Geometry check sheet. Reference: the model listing, model coordinates, mm. A direction names the side the tool comes from. Give positions to 0.01 mm unless a question says otherwise; leave off trailing zeros. Loops run counter-clockwise (first coordinate to the right, second up) from the corner with the lowest first, then second, coordinate; pieces in that order, holes last. Notation, with made-up numbers: (81.25, -6) -> (106.25, -6) arc R23 ccw to (106.25, 15) -> close; hole circle Ø10 at (71, -16.5). An arc over 180 degrees is marked (long way). Answer as a JSON object with one key per item and string values.
from build123d import *

# Parameters (mm, degrees)
EXTRUDE_1_DEPTH     = 60
SKETCH_2_W          = 50
SKETCH_2_H          = 85
CUT_EXTRUDE_1_DEPTH = 70
SKETCH_3_R          = 10
CUT_EXTRUDE_2_DEPTH = 105.880884817
SKETCH_4_R          = 27.5
CUT_EXTRUDE_3_DEPTH = 107.066017178


with BuildPart() as part:
    # Эскиз1 → Бобышка-Вытянуть1 (new, symmetric)
    with BuildSketch(Plane.XY):
        Polygon((50, -25), (0, 45), (-25, 45), (-25, -25), (-50, -25), (-50, -45), (50, -45), align=None)
    extrude(amount=EXTRUDE_1_DEPTH, both=True)

    # Эскиз2 → Вырез-Вытянуть1 (cut)
    with BuildSketch(Plane(origin=(0, 45, 0), x_dir=(1, 0, 0), z_dir=(0, 1, 0))):
        with Locations((25, 0)):
            Rectangle(SKETCH_2_W, SKETCH_2_H)
    extrude(amount=-CUT_EXTRUDE_1_DEPTH, mode=Mode.SUBTRACT)

    # Эскиз3 → Вырез-Вытянуть2 (cut, through all)
    with BuildSketch(Plane(origin=(0, -25, 0), x_dir=(1, 0, 0), z_dir=(0, 1, 0))):
        with Locations(Location((25, 0, 0), (0, 0, 180))):
            Circle(SKETCH_3_R)
    extrude(amount=-CUT_EXTRUDE_2_DEPTH, mode=Mode.SUBTRACT)

    # Эскиз4 → Вырез-Вытянуть3 (cut, through all)
    with BuildSketch(Plane.ZY.offset(25)):
        with Locations((0, 45)):
            Circle(SKETCH_4_R)
    extrude(amount=-CUT_EXTRUDE_3_DEPTH, mode=Mode.SUBTRACT)


solid = part.part
1) Section check B-B on z = 0. Record the cut outline in (x, y), plus the area to 3 significant figures.
Geometry check:
{"outline": "(-50, -45) -> (15, -45) -> (15, -25) -> (0, -25) -> (0, 17.5) -> (-25, 17.5) -> (-25, -25) -> (-50, -25) -> close; (35, -45) -> (50, -45) -> (50, -25) -> (35, -25) -> close", "area": "2,660 mm2"}
2) Depth check by flat-ended pin: P1, Ø6, axis at y = -14.5, z = -47.5, coming from the -X side; P2, Ø6, axis at x = -10.5, z = 5.5, coming from the +Y side; P3, Ø8, axis at y = 18, z = -19, coming from the +X side. Enter the tip coordinate at first touch or a pass-through.
Geometry check:
{"P1": "stops at x = -25", "P2": "stops at y = 18.85", "P3": "stops at x = 0"}
3) Section check D-D on z = -49. Record the cut outline in (x, y).
Geometry check:
{"outline": "(-50, -45) -> (50, -45) -> (50, -25) -> (0, 45) -> (-25, 45) -> (-25, -25) -> (-50, -25) -> close"}
4) Section check A-A on x = 25. Record the cut outline in (y, z), plus the area to 4 significant figures.
Geometry check:
{"outline": "(-45, -60) -> (10, -60) -> (10, -42.5) -> (-25, -42.5) -> (-25, -10) -> (-45, -10) -> close; (-45, 10) -> (-25, 10) -> (-25, 42.5) -> (10, 42.5) -> (10, 60) -> (-45, 60) -> close", "area": "3,225 mm2"}
5) Section check C-C on y = -35.5. Record the cut outline in (x, z), plus the area to 3 significant figures.
Geometry check:
{"outline": "(-50, -60) -> (50, -60) -> (50, 60) -> (-50, 60) -> close; hole circle Ø20 at (25, 0)", "area": "11,700 mm2"}
6) Material ranges on line 1 along Z through (x, y) = (25, -31); line 2 along Z through (x, y) = (27, -7.5); line 3 along Y through (x, z) = (37.5, -9.5), recorded low to high. Write a range as from..to.
Geometry check:
{"line 1": "z = -60..-10, 10..60", "line 2": "z = -60..-42.5, 42.5..60", "line 3": "y = -45..-25"}
7) Tool access check on faces 5 (the face through (-12, 45, -44)), 6 (the face through (-25, 10, 1)), 7 (the face through (0, 3, 1)). Record the directions out of +Z, -Z, +X, -X, +Y, -Y that give a thin tool (end or side, any length) a straight path to the whole face; none if there is none.
Geometry check:
{"face 5": "+Z, -Z, +X, -X, +Y", "face 6": "+Z, -Z, -X, +Y", "face 7": "+X, +Y"}
8) Draft check along Z on faces 1 (the face through (-1, -9, 60)), 2 (the face through (-12, 45, 44)), 3 (the face through (14, -5, 42.5)), 4 (the face through (15.46, -34.86, 3)). Enter one of: pulls with the +Z half, pulls with the -Z half, needs draft (parallel to the pull), parting line crosses it, or undercut.
Geometry check:
{"face 1": "pulls with the +Z half", "face 2": "needs draft", "face 3": "undercut", "face 4": "undercut"}
